Part model, mm, in its own coordinate system. Coordinates: 2 decimals unless noted, no trailing zeros. Order: outer loops, then holes, each group sorted by start corner. A loop starts at its lowest first (then second) coordinate and runs counter-clockwise, first axis right, second up.
1) Cut at A-A (z = 0). List the corners of the cut face in (x, y), and give its area (3 significant figures).
2) Cut at C-C (y = 3.5). List the corners of the cut face in (x, z).
3) Cut at B-B (x = 0). List the corners of the cut face in (y, z).
4) Cut at D-D (y = 0.5). List the corners of the cut face in (x, z), and give its area (3 significant figures).
5) Pin check, flat tips, straight feed: pin 1 Ø1.5 at (x, y) = (-7.5, 1.5) entering from -Z; pin 2 Ø1 at (x, y) = (-5.5, 5) entering from -Z. Stop position of each tip, or through.
6) Mould opens along X. For faces 1 (the conical face through (2.96, 3.13, -0.93)), 2 (the flat face through (-9.075, 3.131, -2.717)), 3 (the flat face through (2.717, 3.131, -9.075)), 4 (the flat face through (4, 0, 0)) say: +X half, -X half, draft (parallel to the pull), parting line (faces both ways), or undercut.
7) Wall check: L1, parallel to Z at x = 0, y = 4.75; L2, parallel to X at y = 5.75, z = -1.25; L3, parallel to X at y = 3, z = 1.5. Give the ranges that are in metal, low to high.
```python
from build123d import *

# Parameters (mm, degrees)
SKETCH1_R           = 3.2385
BOSS_EXTRUDE1_DEPTH = 6.35
BOSS_EXTRUDE1_DRAFT = -2.5


with BuildPart() as part:
    # Sketch1 → Boss-Extrude1 (with draft: the straight prism first)
    with BuildSketch(Plane(origin=(0, 0, 0), x_dir=(1, 0, 0), z_dir=(0, 1, 0))):
        Polygon((8.24563965, -5.042609025), (9.662237919, -0.244207692), (8.489847342, 4.619628895), (5.042609025, 8.24563965), (0.244207692, 9.662237919), (-4.619628895, 8.489847342), (-8.24563965, 5.042609025), (-9.662237919, 0.244207692), (-8.489847342, -4.619628895), (-5.042609025, -8.24563965), (-0.244207692, -9.662237919), (4.619628895, -8.489847342), align=None)
        Circle(SKETCH1_R, mode=Mode.SUBTRACT)
    extrude(amount=BOSS_EXTRUDE1_DEPTH)
    # Boss-Extrude1: the draft: its side faces are tilted about the plane it starts from
    boss_extrude1_sides = [part.faces().sort_by_distance(p)[0] for p in [
        (8.953938785, 3.175, 2.643408358),
        (9.07604263, 3.175, -2.187710601),
        (6.766228183, 3.175, -6.432634272),
        (2.643408358, 3.175, -8.953938785),
        (-2.187710601, 3.175, -9.07604263),
        (-6.432634272, 3.175, -6.766228183),
        (-8.953938785, 3.175, -2.643408358),
        (-9.07604263, 3.175, 2.187710601),
        (-6.766228183, 3.175, 6.432634272),
        (-2.643408358, 3.175, 8.953938785),
        (2.187710601, 3.175, 9.07604263),
        (6.432634272, 3.175, 6.766228183),
        (-3.2385, 3.175, 0),
    ]]
    draft(boss_extrude1_sides, Plane(origin=(0, 0, 0), x_dir=(1, 0, 0), z_dir=(0, 1, 0)), BOSS_EXTRUDE1_DRAFT)


solid = part.part
```
Geometry check:
1. outline: (-9.89, 6.35) - (-9.6, 0) - (-3.24, 0) - (-2.96, 6.35) - close; (2.96, 6.35) - (3.24, 0) - (9.6, 0) - (9.89, 6.35) - close
1. area: 84.4 mm2
2. outline: (-9.82, -0.25) - (-8.38, -5.13) - (-4.7, -8.63) - (0.25, -9.82) - (5.13, -8.38) - (8.63, -4.7) - (9.82, 0.25) - (8.38, 5.13) - (4.7, 8.63) - (-0.25, 9.82) - (-5.13, 8.38) - (-8.63, 4.7) - close; hole circle Ø6.17 at (0, 0)
3. outline: (0, -9.6) - (6.35, -9.89) - (6.35, -2.96) - (0, -3.24) - close; (0, 3.24) - (6.35, 2.96) - (6.35, 9.89) - (0, 9.6) - close
4. outline: (-9.68, -0.24) - (-8.26, -5.05) - (-4.63, -8.51) - (0.24, -9.68) - (5.05, -8.26) - (8.51, -4.63) - (9.68, 0.24) - (8.26, 5.05) - (4.63, 8.51) - (-0.24, 9.68) - (-5.05, 8.26) - (-8.51, 4.63) - close; hole circle Ø6.43 at (0, 0)
4. area: 249 mm2
5. pin 1: stops at z = -6.56
5. pin 2: stops at z = -8.43
6. face 1: undercut
6. face 2: -X half
6. face 3: +X half
6. face 4: draft
7. L1: z = -9.82 to -3.03, 3.03 to 9.82
7. L2: x = -9.63 to -2.71, 2.71 to 9.56
7. L3: x = -9.38 to -2.72, 2.72 to 9.43
